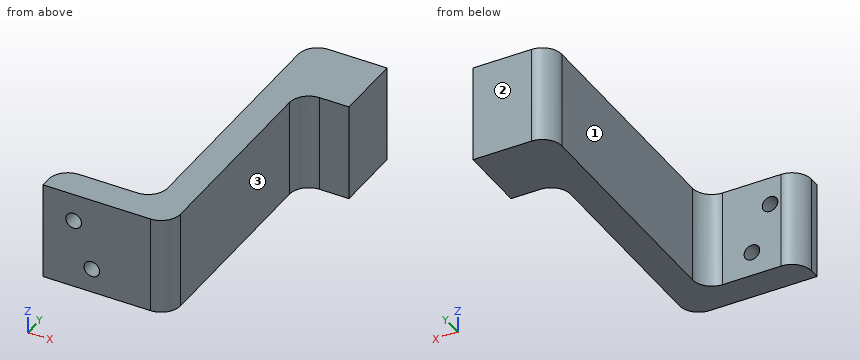
from build123d import *

# Parameters (mm, degrees)
SKETCH1_W                  = 2.5
SKETCH1_H                  = 0.75
BOSS_EXTRUDE1_DEPTH        = 1.875
BOSS_EXTRUDE1_DEPTH_BACK   = 0.625
FILLET1_R                  = 0.5
F_0_4_0_4_DIAMETER_HOLE1_D = 0.4


with BuildPart() as part:
    # Sketch1 → Boss-Extrude1 (new body, two sides)
    with BuildSketch(Plane.XY) as boss_extrude1_sk:
        Polygon((0.285769435, 0.25), (-0.464230565, 0.25), (-0.464230565, -5), (-0.464230565, -5.75), (0.285769435, -5.75), align=None)
        Polygon((-0.464230565, 2), (-0.464230565, 0.25), (0.285769435, 0.25), (1.535769435, 0.25), (1.535769435, 2), align=None)
        with Locations((-1.714230565, -5.375)):
            Rectangle(SKETCH1_W, SKETCH1_H)
    extrude(amount=BOSS_EXTRUDE1_DEPTH)
    extrude(boss_extrude1_sk.sketch, amount=-BOSS_EXTRUDE1_DEPTH_BACK)

    # Fillet1
    fillet1_edges = [part.edges().sort_by_distance(p)[0] for p in [
        (0.285769435, 0.25, 0.625),
        (-2.964230565, -5, 0.625),
        (-0.464230565, -5, 0.625),
        (0.285769435, -5.75, 0.625),
        (-0.464230565, 2, 0.625),
    ]]
    fillet(fillet1_edges, radius=FILLET1_R)

    # Ø0.4 (0.4) Diameter Hole1 (through all)
    with Locations(Plane(origin=(0, -5, 0), x_dir=(1, 0, 0), z_dir=(0, 1, 0))):
        with Locations((-1.714230565, 0), (-2.17846891, -1.160595864)):
            Hole(F_0_4_0_4_DIAMETER_HOLE1_D / 2)


solid = part.part
CAD build for the part. Positions are in the model's coordinates, mm. Face numbers are marked on the shaded views. A direction names the side the tool comes from. Coordinates: 2 decimals unless noted, no trailing zeros. Order: outer loops, then holes, each group sorted by start corner. A loop starts at its lowest first (then second) coordinate and runs counter-clockwise, first axis right, second up.
Item 1: Band-saw the part on D-D on y = 1. List the corners of the cut face in (x, z) (3 decimals).
Check sheet entries:
outline: (-0.464, -0.625) - (1.536, -0.625) - (1.536, 1.875) - (-0.464, 1.875) - close
Item 2: Band-saw the part on C-C on z = 0.7. List the corners of the cut face in (x, y).
Check sheet entries:
outline: (-2.96, -5.75) - (-0.21, -5.75) arc R0.5 ccw to (0.29, -5.25) - (0.29, -0.25) arc R0.5 cw to (0.79, 0.25) - (1.54, 0.25) - (1.54, 2) - (0.04, 2) arc R0.5 ccw to (-0.46, 1.5) - (-0.46, -4.5) arc R0.5 cw to (-0.96, -5) - (-2.46, -5) arc R0.5 ccw to (-2.96, -5.5) - close
Item 3: Drill centre lines: L1, parallel to X at y = -2, z = 0.2; L2, parallel to Y at x = 1.15, z = 0.8; L3, parallel to Y at x = -1.4, z = 1.1. Where is each one in solid material? Low to high.
Check sheet entries:
L1: x = -0.46 to 0.29
L2: y = 0.25 to 2
L3: y = -5.75 to -5
Item 4: 3-axis set-ups, long thin cutter, end or side, ignore diameter. For the marked faces 1, 2 and 3: which of +Z, -Z, +X, -X, +Y, -Y reach the whole face in a straight line?
Check sheet entries:
face 1: +Z, -Z, -X, +Y
face 2: +Z, -Z, +X, -X, +Y
face 3: +Z, -Z, +X, -Y
Item 5: Band-saw the part on B-B on x = -2.15. List the corners of the cut face in (y, z) (3 decimals).
Check sheet entries:
outline: (-5.75, -0.625) - (-5, -0.625) - (-5, 0.963) - (-5.75, 0.963) - close; (-5.75, 1.359) - (-5, 1.359) - (-5, 1.875) - (-5.75, 1.875) - close
Item 6: Pin check, flat tips, straight feed: pin 1 Ø0.8 at (x, z) = (-1.5, 0.5) entering from +Y; pin 2 Ø1 at (y, z) = (-3.5, 1.5) entering from -X. Stop position of each tip, or through.
Check sheet entries:
pin 1: stops at y = -5
pin 2: stops at x = -0.46
Item 7: Band-saw the part on A-A on z = 0. List the corners of the cut face in (x, y).
Check sheet entries:
outline: (-2.96, -5.75) - (-1.91, -5.75) - (-1.91, -5) - (-2.46, -5) arc R0.5 ccw to (-2.96, -5.5) - close; (-1.51, -5.75) - (-0.21, -5.75) arc R0.5 ccw to (0.29, -5.25) - (0.29, -0.25) arc R0.5 cw to (0.79, 0.25) - (1.54, 0.25) - (1.54, 2) - (0.04, 2) arc R0.5 ccw to (-0.46, 1.5) - (-0.46, -4.5) arc R0.5 cw to (-0.96, -5) - (-1.51, -5) - close
